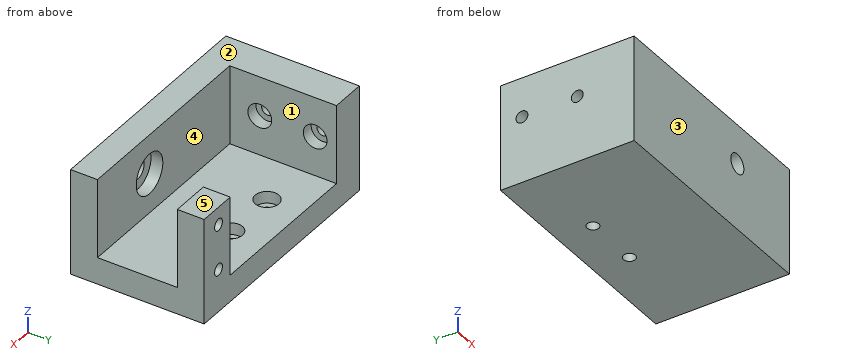
from build123d import *

# Parameters (mm, degrees)
BOSS_EXTRUDE2_DEPTH  = 20
SKETCH4_W            = 6.8
SKETCH4_H            = 33.8
BOSS_EXTRUDE3_DEPTH  = 53.6
SKETCH8_W            = 20
SKETCH8_H            = 20.2
CUT_EXTRUDE1_DEPTH   = 53.6
SKETCH9_R            = 5
CUT_EXTRUDE3_DEPTH   = 3
SKETCH11_R           = 2.5
CUT_EXTRUDE4_DEPTH   = 20
SKETCH12_R           = 1.1
CUT_EXTRUDE6_DEPTH   = 20
SKETCH13_W           = 2
SKETCH13_H           = 26.8
BOSS_EXTRUDE4_DEPTH  = 33.8
SKETCH16_R           = 1.1
CUT_EXTRUDE7_DEPTH   = 20
SKETCH17_W           = 2
SKETCH17_H           = 26.8
BOSS_EXTRUDE5_DEPTH  = 33.8
SKETCH18_W           = 20
SKETCH18_H           = 20.2
CUT_EXTRUDE9_DEPTH   = 60
SKETCH19_W           = 20
SKETCH19_H           = 20.2
CUT_EXTRUDE10_DEPTH  = 60
SKETCH20_W           = 8.8
SKETCH20_H           = 20.2
BOSS_EXTRUDE6_DEPTH  = 20
SKETCH21_R           = 1.1
BOSS_EXTRUDE7_DEPTH  = 13.6
SKETCH23_R           = 1.1
BOSS_EXTRUDE8_DEPTH  = 13.6
SKETCH24_R           = 1.125173923
BOSS_EXTRUDE9_DEPTH  = 6.8
SKETCH25_R           = 1.1
SKETCH25_R_2         = 1.440897936
BOSS_EXTRUDE10_DEPTH = 6.8
SKETCH26_R           = 1.5
CUT_EXTRUDE11_DEPTH  = 10
SKETCH27_R           = 1.5
CUT_EXTRUDE12_DEPTH  = 10
SKETCH29_R           = 1.5
CUT_EXTRUDE15_DEPTH  = 10
SKETCH31_R           = 3
CUT_EXTRUDE16_DEPTH  = 3
SKETCH32_R           = 3
CUT_EXTRUDE17_DEPTH  = 3
SKETCH33_R           = 5.1
CUT_EXTRUDE18_DEPTH  = 3
SKETCH35_W           = 6.8
SKETCH35_H           = 20.2
BOSS_EXTRUDE11_DEPTH = 2
SKETCH36_R           = 2.5
BOSS_EXTRUDE13_DEPTH = 6.8
SKETCH37_R           = 1.5
CUT_EXTRUDE19_DEPTH  = 6.8


with BuildPart() as part:
    # Sketch1 → Boss-Extrude2 (new body)
    with BuildSketch(Plane.XY):
        Polygon((-13.090120482, -4.867831325), (27.713257426, -4.867831325), (27.713257426, 21.982168675), (34.513257426, 21.982168675), (34.513257426, -5.017831325), (34.513257426, -11.817831325), (-19.890120482, -11.817831325), (-19.890120482, -5.017831325), (-19.890120482, 21.982168675), (-13.090120482, 21.982168675), align=None)
    extrude(amount=BOSS_EXTRUDE2_DEPTH)

    # Sketch4 → Boss-Extrude3 (add)
    with BuildSketch(Plane.ZY.offset(19.890120482)):
        with Locations((-3.4, 5.082168675)):
            Rectangle(SKETCH4_W, SKETCH4_H)
    extrude(amount=-BOSS_EXTRUDE3_DEPTH)

    # Sketch8 → Cut-Extrude1 (cut)
    with BuildSketch(Plane(origin=(34.513257426, 0, 0), x_dir=(0, 0, -1), z_dir=(1, 0, 0))):
        with Locations((-10, 5.082168675)):
            Rectangle(SKETCH8_W, SKETCH8_H)
    extrude(amount=-CUT_EXTRUDE1_DEPTH, mode=Mode.SUBTRACT)

    # Sketch9 → Cut-Extrude3 (cut)
    with BuildSketch(Plane(origin=(0, -5.017831325, 0), x_dir=(1, 0, 0), z_dir=(0, 1, 0))):
        with Locations(Location((17.713257426, -10, 0), (0, 0, 270))):
            Circle(SKETCH9_R)
    extrude(amount=-CUT_EXTRUDE3_DEPTH, mode=Mode.SUBTRACT)

    # Sketch11 → Cut-Extrude4 (cut)
    with BuildSketch(Plane(origin=(0, -8.017831325, 0), x_dir=(1, 0, 0), z_dir=(0, 1, 0))):
        with Locations(Location((17.713257426, -10, 0), (0, 0, 270))):
            Circle(SKETCH11_R)
    extrude(amount=-CUT_EXTRUDE4_DEPTH, mode=Mode.SUBTRACT)

    # Sketch12 → Cut-Extrude6 (cut)
    with BuildSketch(Plane(origin=(0, 21.982168675, 0), x_dir=(1, 0, 0), z_dir=(0, 1, 0))):
        with Locations(Location((32.513257426, -15.3, 0), (0, 0, 180))):
            Circle(SKETCH12_R)
        with Locations(Location((31.709879518, -4.7, 0), (0, 0, 180))):
            Circle(SKETCH12_R)
    extrude(amount=-CUT_EXTRUDE6_DEPTH, mode=Mode.SUBTRACT)

    # Sketch13 → Boss-Extrude4 (add)
    with BuildSketch(Plane(origin=(0, 21.982168675, 0), x_dir=(1, 0, 0), z_dir=(0, 1, 0))):
        with Locations((34.709879518, -6.6)):
            Rectangle(SKETCH13_W, SKETCH13_H)
    extrude(amount=-BOSS_EXTRUDE4_DEPTH)

    # Sketch16 → Cut-Extrude7 (cut)
    with BuildSketch(Plane(origin=(0, 21.982168675, 0), x_dir=(1, 0, 0), z_dir=(0, 1, 0))):
        with Locations(Location((-17.890120482, -15.3, 0), (0, 0, 180))):
            Circle(SKETCH16_R)
        with Locations(Location((-17.890120482, -4.7, 0), (0, 0, 180))):
            Circle(SKETCH16_R)
    extrude(amount=-CUT_EXTRUDE7_DEPTH, mode=Mode.SUBTRACT)

    # Sketch17 → Boss-Extrude5 (add)
    with BuildSketch(Plane(origin=(0, 21.982168675, 0), x_dir=(1, 0, 0), z_dir=(0, 1, 0))):
        with Locations((-20.890120482, -6.6)):
            Rectangle(SKETCH17_W, SKETCH17_H)
    extrude(amount=-BOSS_EXTRUDE5_DEPTH)

    # Sketch18 → Cut-Extrude9 (cut)
    with BuildSketch(Plane.ZY.offset(-33.709879518)):
        with Locations((10, 5.082168675)):
            Rectangle(SKETCH18_W, SKETCH18_H)
    extrude(amount=CUT_EXTRUDE9_DEPTH, mode=Mode.SUBTRACT)

    # Sketch19 → Cut-Extrude10 (cut)
    with BuildSketch(Plane.ZY.offset(-33.709879518)):
        with Locations((10, 5.082168675)):
            Rectangle(SKETCH19_W, SKETCH19_H)
    extrude(amount=-CUT_EXTRUDE10_DEPTH, mode=Mode.SUBTRACT)

    # Sketch20 → Boss-Extrude6 (add)
    with BuildSketch(Plane.XY):
        with Locations((-17.490120482, 5.082168675)):
            Rectangle(SKETCH20_W, SKETCH20_H)
    extrude(amount=BOSS_EXTRUDE6_DEPTH)

    # Sketch21 → Boss-Extrude7 (add)
    with BuildSketch(Plane(origin=(0, 21.982168675, 0), x_dir=(1, 0, 0), z_dir=(0, 1, 0))):
        with Locations((-17.890120482, -4.7)):
            Circle(SKETCH21_R)
    extrude(amount=-BOSS_EXTRUDE7_DEPTH)

    # Sketch23 → Boss-Extrude8 (add)
    with BuildSketch(Plane(origin=(0, 21.982168675, 0), x_dir=(1, 0, 0), z_dir=(0, 1, 0))):
        with Locations((-17.890120482, -15.3)):
            Circle(SKETCH23_R)
    extrude(amount=-BOSS_EXTRUDE8_DEPTH)

    # Sketch24 → Boss-Extrude9 (add)
    with BuildSketch(Plane(origin=(0, 21.982168675, 0), x_dir=(1, 0, 0), z_dir=(0, 1, 0))):
        with Locations((32.513257426, -15.3)):
            Circle(SKETCH24_R)
    extrude(amount=-BOSS_EXTRUDE9_DEPTH)

    # Sketch25 → Boss-Extrude10 (add)
    with BuildSketch(Plane(origin=(0, 21.982168675, 0), x_dir=(1, 0, 0), z_dir=(0, 1, 0))):
        with Locations((29.715206423, -15.150513528)):
            Circle(SKETCH25_R)
        with Locations((31.709879518, -4.7)):
            Circle(SKETCH25_R_2)
    extrude(amount=-BOSS_EXTRUDE10_DEPTH)

    # Sketch26 → Cut-Extrude11 (cut)
    with BuildSketch(Plane(origin=(0, 21.982168675, 0), x_dir=(1, 0, 0), z_dir=(0, 1, 0))):
        with Locations(Location((32.213257426, -4.5, 0), (0, 0, 180))):
            Circle(SKETCH26_R)
        with Locations(Location((32.213257426, -15.5, 0), (0, 0, 180))):
            Circle(SKETCH26_R)
    extrude(amount=-CUT_EXTRUDE11_DEPTH, mode=Mode.SUBTRACT)

    # Sketch27 → Cut-Extrude12 (cut)
    with BuildSketch(Plane(origin=(0, 0, -6.8), x_dir=(-1, 0, 0), z_dir=(0, 0, -1))):
        with Locations(Location((-13.909879518, 12.982168675, 0), (0, 0, 90))):
            Circle(SKETCH27_R)
        with Locations(Location((0.090120482, 12.982168675, 0), (0, 0, 90))):
            Circle(SKETCH27_R)
    extrude(amount=-CUT_EXTRUDE12_DEPTH, mode=Mode.SUBTRACT)

    # Sketch29 → Cut-Extrude15 (cut)
    with BuildSketch(Plane.ZY.offset(21.890120482)):
        with Locations(Location((10, 2.582168675, 0), (0, 0, 270))):
            Circle(SKETCH29_R)
        with Locations(Location((10, 16.582168675, 0), (0, 0, 270))):
            Circle(SKETCH29_R)
    extrude(amount=-CUT_EXTRUDE15_DEPTH, mode=Mode.SUBTRACT)

    # Sketch31 → Cut-Extrude16 (cut)
    with BuildSketch(Plane(origin=(-13.090120482, 0, 0), x_dir=(0, 0, -1), z_dir=(1, 0, 0))):
        with Locations(Location((-10, 2.582168675, 0), (0, 0, 90))):
            Circle(SKETCH31_R)
        with Locations(Location((-10, 16.582168675, 0), (0, 0, 90))):
            Circle(SKETCH31_R)
    extrude(amount=-CUT_EXTRUDE16_DEPTH, mode=Mode.SUBTRACT)

    # Sketch32 → Cut-Extrude17 (cut)
    with BuildSketch(Plane.XY):
        with Locations((-0.090120482, 12.982168675)):
            Circle(SKETCH32_R)
        with Locations((13.909879518, 12.982168675)):
            Circle(SKETCH32_R)
    extrude(amount=-CUT_EXTRUDE17_DEPTH, mode=Mode.SUBTRACT)

    # Sketch33 → Cut-Extrude18 (cut)
    with BuildSketch(Plane(origin=(0, -5.017831325, 0), x_dir=(1, 0, 0), z_dir=(0, 1, 0))):
        with Locations(Location((17.713257426, -10, 0), (0, 0, 270))):
            Circle(SKETCH33_R)
    extrude(amount=-CUT_EXTRUDE18_DEPTH, mode=Mode.SUBTRACT)

    # Sketch35 → Boss-Extrude11 (add)
    with BuildSketch(Plane(origin=(35.709879518, 0, 0), x_dir=(0, 0, -1), z_dir=(1, 0, 0))):
        Polygon((-20, 21.982168675), (-20, 15.182168675), (0, 15.182168675), (6.8, 15.182168675), (6.8, 21.982168675), align=None)
        with Locations((3.4, 5.082168675)):
            Rectangle(SKETCH35_W, SKETCH35_H)
        Polygon((6.8, -5.017831325), (0, -5.017831325), (-20, -5.017831325), (-20, -11.817831325), (6.8, -11.817831325), align=None)
    extrude(amount=BOSS_EXTRUDE11_DEPTH)

    # Sketch36 → Boss-Extrude13 (add)
    with BuildSketch(Plane(origin=(0, 21.982168675, 0), x_dir=(1, 0, 0), z_dir=(0, 1, 0))):
        with Locations((31.713257426, -4)):
            Circle(SKETCH36_R)
    extrude(amount=-BOSS_EXTRUDE13_DEPTH)

    # Sketch37 → Cut-Extrude19 (cut)
    with BuildSketch(Plane(origin=(0, 21.982168675, 0), x_dir=(1, 0, 0), z_dir=(0, 1, 0))):
        with Locations(Location((32.213257426, -4, 0), (0, 0, 180))):
            Circle(SKETCH37_R)
    extrude(amount=-CUT_EXTRUDE19_DEPTH, mode=Mode.SUBTRACT)


solid = part.part
Geometry check sheet. Reference: the model listing, model coordinates, mm. Face numbers are marked on the shaded views. A direction names the side the tool comes from. Coordinates: 2 decimals unless noted, no trailing zeros. Order: outer loops, then holes, each group sorted by start corner. A loop starts at its lowest first (then second) coordinate and runs counter-clockwise, first axis right, second up. Notation, with made-up numbers: (-27, 30.25) -> (-16, 30.25) arc R30 cw to (-16, 64.25) -> close; hole circle Ø5 at (39, 38.25). An arc over 180 degrees is marked (long way). Use a Markdown table: item, result. Add a question column.
1. Cross-section at A-A (z = 0.75). Enter the section's corners in (x, y).
2. Material ranges on L1, parallel to Y at x = 34.5, z = 13.75; L2, parallel to X at y = 19.5, z = 5; L3, parallel to Y at x = -16, z = 11, recorded low to high.
3. Cross-section at B-B (z = 10). Give the number of separate pieces and of enclosed holes in the cut face, and give its area (3 significant figures).
4. Cross-section at C-C (x = 30). Enter the section's corners in (y, z), and give its area (3 significant figures).
5. Go/stop test with flat-tipped pins: pin 1 Ø11 at (x, z) = (19.5, 12.5) entering from +Y; pin 2 Ø4 at (x, y) = (13.91, 12.98) entering from +Z; pin 3 Ø1 at (x, y) = (24.5, -4) entering from +Z. Record where each tip stops, or that it passes through.
6. Mould release check, pull along Y, two halves, no side actions. Record for the marked faces 3, 4 and 5: pulls with the +Y half, pulls with the -Y half, needs draft (parallel to the pull), parting line crosses it, or undercut.
7. Set-up check for the marked faces 1 and 2: record each of +Z, -Z, +X, -X, +Y, -Y from which the full face is reachable in a straight line by a thin tool's end or side.
8. Cross-section at D-D (z = 4). Enter the section's corners in (x, y), and give its area (3 significant figures).
Filled sheet:
| question | item | result |
|---|---|---|
| 1 | outline | (-21.89, -11.82) -> (37.71, -11.82) -> (37.71, -5.02) -> (-13.09, -5.02) -> (-13.09, 21.98) -> (-21.89, 21.98) -> close; (27.71, 15.18) -> (37.71, 15.18) -> (37.71, 21.98) -> (27.71, 21.98) -> close |
| 2 | L1 | -11.82 to -5.02, 15.18 to 21.98 |
| 2 | L2 | -21.89 to -13.09, 27.71 to 31.1, 33.33 to 37.71 |
| 2 | L3 | -11.82 to -0.25, 5.41 to 13.75, 19.41 to 21.98 |
| 3 | separate pieces | 5 |
| 3 | enclosed holes | 0 |
| 3 | area | 590 mm2 |
| 4 | outline | (-11.82, -6.8) -> (21.98, -6.8) -> (21.98, 20) -> (15.18, 20) -> (15.18, 0) -> (-5.02, 0) -> (-5.02, 20) -> (-11.82, 20) -> close |
| 4 | area | 502 mm2 |
| 5 | pin 1 | y = -5.02 |
| 5 | pin 2 | z = -3 |
| 5 | pin 3 | z = 0 |
| 6 | face 3 | pulls with the -Y half |
| 6 | face 4 | undercut |
| 6 | face 5 | needs draft |
| 7 | face 1 | +Z, +Y |
| 7 | face 2 | +Z, +X, -X, +Y, -Y |
| 8 | outline | (-21.89, -11.82) -> (37.71, -11.82) -> (37.71, -5.02) -> (-13.09, -5.02) -> (-13.09, 21.98) -> (-21.89, 21.98) -> close; (27.71, 15.18) -> (30.71, 15.18) -> (30.71, 21.98) -> (27.71, 21.98) -> close; (33.71, 15.18) -> (37.71, 15.18) -> (37.71, 21.98) -> (33.71, 21.98) -> close |
| 8 | area | 690 mm2 |
